Autodesk Inventor part; units mm, degrees
ref_plane "YZ Plane" through (0, 0, 0) normal (1, 0, 0) x (0, 1, 0)
ref_plane "XZ Plane" through (0, 0, 0) normal (0, 1, 0) x (-1, 0, 0)
ref_plane "XY Plane" through (0, 0, 0) normal (0, 0, 1) x (1, 0, 0)
sketch "Sketch1" plane through (0, 0, 0) normal (0, 0, 1) x (1, 0, 0)
  circle A0 centre (0, 0) radius 18.5
  circle A1 centre (0, 0) radius 24.125
  circle A2 centre (0, 0) radius 25.4
  circle A3 centre (0, 0) radius 18
  point P0 (-21, 0)
  point P1 (21, 0)
  dimension "d" = 37
  dimension "d1" = 48.25
  dimension "d2" = 50.8
  dimension "d14" = 21
  dimension "d15" = 21
  dimension "d16" = 36
extrude "Extrusion1" add sketch "Sketch1" along normal blind 5.5 contours A1
extrude "Extrusion2" add sketch "Sketch1" along normal blind 1 contours A2
hole "Hole1" at (-21, 0, 0) at (21, 0, 0) direction (0, 0, 1) diameter 2 end through all
extrude "Extrusion3" add sketch "Sketch1" along normal blind 1 contours A0
properties part number "Adapter-D37mm-SM2"
Design review of the part built by this model. Coordinates are the model's own, in mm. A direction names the side the tool comes from. Give positions to 0.01 mm unless a question says otherwise; leave off trailing zeros. Write each loop counter-clockwise with the first axis right and the second up, starting at its lowest first coordinate (ties: lowest second). Pieces come first, ordered by that corner, then holes. Notation, with made-up numbers: (23.25, 40.5) - (32.25, 40.5) arc R13 ccw to (32.25, 56.5) - close; hole circle Ø8 at (47, -10.5). An arc over 180 degrees is marked (long way). Return JSON: item names as keys, results as strings. Group by question number.
(1) We need section C-C, the plane y = 11. Give the boundary of the cut face in (x, z), then the cut area to 3 significant figures.
(2) We need section A-A, the plane y = 0. Give the boundary of the cut face in (x, z) (3 decimals), then the cut area to 3 significant figures.
(3) We need section B-B, the plane x = 0. Give the boundary of the cut face in (y, z) (3 decimals), then the cut area to 3 significant figures.
(4) Insertion check: pin 1 (3 mm diameter, centred on x = -20, z = 3.5, fed in from +Y); pin 2 (2.5 mm diameter, centred on x = -21, y = 0, fed in from -Z); pin 3 (1 mm diameter, centred on y = 13, z = 1, fed in from -X). Each pin has a flat end and moves straight along its axis. Give the tip position at first contact, or say it passes through.
(5) Machinability: for faces 4 (the cylindrical face through (-5.506, 24.796, 0.493)), 5 (the flat face through (22.5, -9.3, 1)), which of the approach directions +Z, -Z, +X, -X, +Y, -Y give a long, thin tool a straight path to every point of the face, cutting with its end or side? Answer none if there is none.
(6) To check wall thickness, follow probe 1 along Y at (x, z) = (0, 3.75) (3 decimals); probe 2 along Y at (x, z) = (0, 0.5); probe 3 along Z at (x, y) = (16, -19.5). State the ranges of each line that lie inside material, in increasing order.
(7) We need section D-D, the plane z = 3.4. Give the boundary of the cut face in (x, y) (3 decimals), then the cut area to 3 significant figures.
(8) Mouldability with a two-part tool opening along Y and no side actions: class faces 1 (the cylindrical face through (-20, 0, 3)), 2 (the cylindrical face through (-24.1, -1.1, 3.2)), 3 (the flat face through (-6, 17.3, 0)) as +Y half, -Y half, draft (parallel to the pull), parting line (faces both ways), or undercut.
Reported:
{
 "1": {"outline": "(-22.89, 0) - (-14.25, 0) - (-14.25, 1) - (-14.87, 1) - (-14.87, 5.5) - (-21.47, 5.5) - (-21.47, 1) - (-22.89, 1) - close; (14.25, 0) - (22.89, 0) - (22.89, 1) - (21.47, 1) - (21.47, 5.5) - (14.87, 5.5) - (14.87, 1) - (14.25, 1) - close", "area": "76.7 mm2"},
 "2": {"outline": "(-25.4, 0) - (-22, 0) - (-22, 5.5) - (-24.125, 5.5) - (-24.125, 1) - (-25.4, 1) - close; (-20, 0) - (-18, 0) - (-18, 1) - (-18.5, 1) - (-18.5, 5.5) - (-20, 5.5) - close; (18, 0) - (20, 0) - (20, 5.5) - (18.5, 5.5) - (18.5, 1) - (18, 1) - close; (22, 0) - (25.4, 0) - (25.4, 1) - (24.125, 1) - (24.125, 5.5) - (22, 5.5) - close", "area": "43.4 mm2"},
 "3": {"outline": "(-25.4, 0) - (-18, 0) - (-18, 1) - (-18.5, 1) - (-18.5, 5.5) - (-24.125, 5.5) - (-24.125, 1) - (-25.4, 1) - close; (18, 0) - (25.4, 0) - (25.4, 1) - (24.125, 1) - (24.125, 5.5) - (18.5, 5.5) - (18.5, 1) - (18, 1) - close", "area": "65.4 mm2"},
 "4": {"pin 1": "stops at y = 15.48", "pin 2": "stops at z = 0", "pin 3": "stops at x = -22.11"},
 "5": {"face 4": "+Z, -Z", "face 5": "+Z"},
 "6": {"probe 1": "y = -24.125 to -18.5, 18.5 to 24.125", "probe 2": "y = -25.4 to -18, 18 to 25.4", "probe 3": "z = 0 to 1"},
 "7": {"outline": "circle Ø48.25 at (0, 0); hole circle Ø2 at (-21, 0); hole circle Ø37 at (0, 0); hole circle Ø2 at (21, 0)", "area": "747 mm2"},
 "8": {"face 1": "undercut", "face 2": "parting line", "face 3": "draft"}
}
